Input: part model. Units: mm. Frame: model coordinates. A direction names the side the tool comes from. Give positions to 0.01 mm unless a question says otherwise; leave off trailing zeros. Answer in a Markdown table with one row per item. Add a question column.
1. Mould query, pull axis Y, two halves, no side actions, for faces 3 (the face through (-8.3, -8, 0)), 4 (the face through (5.19, -9.98, 3.45)), 5 (the face through (-23.8, 4.85, 6.4)), 6 (the face through (4.67, -13.2, 3.48)). Classes: released by +Y, released by -Y, zero draft, split by the parting line, or undercut.
2. Access query for faces 1 (the face through (-27, 0, 3)), 2 (the face through (13.2, 4.67, 3.48)). Directions: +Z, -Z, +X, -X, +Y, -Y. A direction counts if a zero-diameter tool reaches every point of the face in a straight line with its end or side. Return the directions, or none.
3. Ray query, line 1 (Y direction, x = 0, z = 1.5); line 2 (Y direction, x = 32, z = 0.75); line 3 (Y direction, x = -35, z = 4.25). Return the intervals inside material, ascending. Write a range as [from, to].
4. Contact query for flat-ended pins moving along their axis: pin 1 (1.5 mm diameter, centred on y = 22, z = 4, fed in from -X); pin 2 (3.5 mm diameter, centred on y = -30.5, z = 3.5, fed in from +X); pin 3 (1.5 mm diameter, centred on y = 2, z = 5, fed in from +X). Output: stop coordinate, or through.
```python
from build123d import *

# Parameters (mm, degrees)
F0_R     = 11.25
F1_DEPTH = 7
F2_R     = 2
F3_R     = 2


with BuildPart() as f1:
    # F0 (on Top) → F1 (new body)
    with BuildSketch(Plane.XY):
        with BuildLine():
            Line((10.8037274316, 8.9039021549), (14, 0))
            ThreePointArc((14, 0), (13.1767253907, 4.7301065505), (10.8037274316, 8.9039021549))
        make_face()
        with BuildLine():
            Line((39, 0), (14, 0))
            ThreePointArc((14, 0), (12.6620422952, -5.97266146), (8.9039021549, -10.8037274316))
            Line((8.9039021549, -10.8037274316), (39, 0))
        make_face()
        with BuildLine():
            ThreePointArc((8.9039021549, -10.8037274316), (12.6620422952, -5.97266146), (14, 0))
            Line((14, 0), (10.8037274316, 8.9039021549))
            ThreePointArc((10.8037274316, 8.9039021549), (5.97266146, 12.6620422952), (0, 14))
            Line((0, 14), (-8.9039021549, 10.8037274316))
            ThreePointArc((-8.9039021549, 10.8037274316), (-12.6620422952, 5.97266146), (-14, 0))
            Line((-14, 0), (-10.8037274316, -8.9039021549))
            ThreePointArc((-10.8037274316, -8.9039021549), (-5.97266146, -12.6620422952), (0, -14))
            Line((0, -14), (8.9039021549, -10.8037274316))
        make_face()
        Circle(F0_R, mode=Mode.SUBTRACT)
        with BuildLine():
            ThreePointArc((0, 14), (5.97266146, 12.6620422952), (10.8037274316, 8.9039021549))
            Line((10.8037274316, 8.9039021549), (0, 39))
            Line((0, 39), (0, 14))
        make_face()
        with BuildLine():
            ThreePointArc((0, -14), (4.7301065505, -13.1767253907), (8.9039021549, -10.8037274316))
            Line((8.9039021549, -10.8037274316), (0, -14))
        make_face()
        with BuildLine():
            Line((-8.9039021549, 10.8037274316), (0, 14))
            ThreePointArc((0, 14), (-4.7301065505, 13.1767253907), (-8.9039021549, 10.8037274316))
        make_face()
        with BuildLine():
            Line((0, -39), (0, -14))
            ThreePointArc((0, -14), (-5.97266146, -12.6620422952), (-10.8037274316, -8.9039021549))
            Line((-10.8037274316, -8.9039021549), (0, -39))
        make_face()
        with BuildLine():
            ThreePointArc((-14, 0), (-12.6620422952, 5.97266146), (-8.9039021549, 10.8037274316))
            Line((-8.9039021549, 10.8037274316), (-39, 0))
            Line((-39, 0), (-14, 0))
        make_face()
        with BuildLine():
            ThreePointArc((-14, 0), (-13.1767253907, -4.7301065505), (-10.8037274316, -8.9039021549))
            Line((-10.8037274316, -8.9039021549), (-14, 0))
        make_face()
    extrude(amount=F1_DEPTH)

    # F2
    f2_edges = [f1.edges().sort_by_distance(p)[0] for p in [
        (0, -26.5, 7),
        (23.951951, -5.401864, 7),
        (5.401864, 23.951951, 7),
        (-23.951951, 5.401864, 7),
        (-26.5, 0, 7),
        (-5.401864, -23.951951, 7),
        (0, 26.5, 7),
        (13.176725, 4.730107, 7),
        (-4.730107, 13.176725, 7),
        (-13.176725, -4.730107, 7),
        (4.730107, -13.176725, 7),
        (26.5, 0, 7),
    ]]
    fillet(f2_edges, radius=F2_R)

    # F3
    f3_edges = [f1.edges().sort_by_distance(p)[0] for p in [
        (-26.5, 0, 0),
        (-5.401864, -23.951951, 0),
        (0, -26.5, 0),
        (23.951951, -5.401864, 0),
        (26.5, 0, 0),
        (5.401864, 23.951951, 0),
        (0, 26.5, 0),
        (-23.951951, 5.401864, 0),
        (4.730107, -13.176725, 0),
        (-13.176725, -4.730107, 0),
        (-4.730107, 13.176725, 0),
        (13.176725, 4.730107, 0),
    ]]
    fillet(f3_edges, radius=F3_R)


solid = f1.part
```
Answer:
| question | item | result |
|---|---|---|
| 1 | face 3 | zero draft |
| 1 | face 4 | undercut |
| 1 | face 5 | released by +Y |
| 1 | face 6 | released by -Y |
| 2 | face 1 | +Z, -Z, -X, -Y |
| 2 | face 2 | +Z, -Z, +X, +Y |
| 3 | line 1 | y = [-13.94, -11.25], [11.25, 13.94] |
| 3 | line 2 | y = [-2.05, -0.44] |
| 3 | line 3 | y = [0, 1.44] |
| 4 | pin 1 | stops at x = 0 |
| 4 | pin 2 | stops at x = 0 |
| 4 | pin 3 | stops at x = 13.94 |
